For this review, take the finished solid that the model builds, in its own axes (mm). Face numbers are marked on the shaded views. A direction names the side the tool comes from. Coordinates: 2 decimals unless noted, no trailing zeros. Write each loop counter-clockwise with the first axis right and the second up, starting at its lowest first coordinate (ties: lowest second). Pieces come first, ordered by that corner, then holes. Notation, with made-up numbers: M 48,32.5 L 55,32.5 A25 cw 55,69.5 Z; hole C 41.5,-37.5 d7. An arc over 180 degrees is marked long. Return JSON: item names as keys, results as strings.
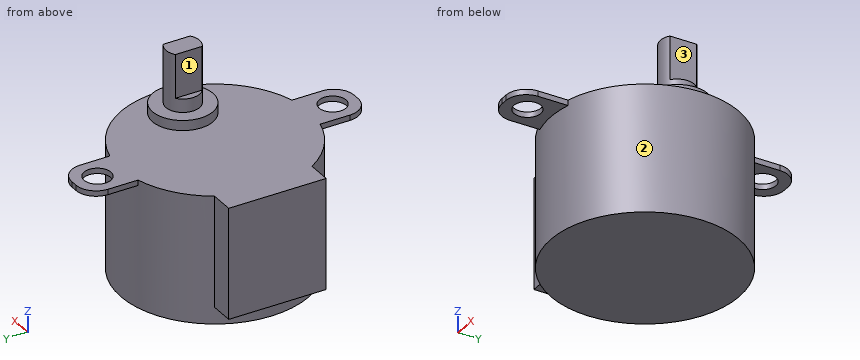
```python
from build123d import *

# Parameters (mm, degrees)
CYLINDER012_R             = 2
CYLINDER012_DEPTH         = 20
CYLINDER011_R             = 2
CYLINDER011_DEPTH         = 20
CYLINDER014_R             = 4.5
CYLINDER014_DEPTH         = 19.5
BOX009_W                  = 7
BOX009_H                  = 42
BOX009_DEPTH              = 0.8
FILLET008_R               = 3
FILLET009_R               = 3
FILLET010_R               = 3
FILLET011_R               = 3
BOX008_W                  = 10
BOX008_H                  = 14.5
BOX008_DEPTH              = 16.5
CYLINDER010_R             = 14
CYLINDER010_DEPTH         = 19
BOX010_W                  = 10
BOX010_H                  = 10
BOX010_DEPTH              = 10
BOX011_W                  = 10
BOX011_H                  = 10
BOX011_DEPTH              = 10
CYLINDER013_R             = 2.5
CYLINDER013_DEPTH         = 28
FUSION011_PLACEMENT_ANGLE = 180


with BuildPart() as cylinder012:
    # Cylinder012 → Cylinder012 (new body)
    with BuildSketch(Plane(origin=(0, -17.5, 14), x_dir=(1, 0, 0), z_dir=(0, 0, 1))):
        Circle(CYLINDER012_R)
    extrude(amount=CYLINDER012_DEPTH)


with BuildPart() as cylinder011:
    # Cylinder011 → Cylinder011 (new body)
    with BuildSketch(Plane(origin=(0, 17.5, 14), x_dir=(1, 0, 0), z_dir=(0, 0, 1))):
        Circle(CYLINDER011_R)
    extrude(amount=CYLINDER011_DEPTH)


with BuildPart() as shaft_boss002:
    # Cylinder014 → Cylinder014 (new body)
    with BuildSketch(Plane(origin=(-8, 0, 1), x_dir=(1, 0, 0), z_dir=(0, 0, 1))):
        Circle(CYLINDER014_R)
    extrude(amount=CYLINDER014_DEPTH)


with BuildPart() as fillet011:
    # Box009 → Box009 (new body)
    with BuildSketch(Plane(origin=(-3.5, -21, 18.2), x_dir=(1, 0, 0), z_dir=(0, 0, 1))):
        with Locations((3.5, 21)):
            Rectangle(BOX009_W, BOX009_H)
    extrude(amount=BOX009_DEPTH)

    # Fillet008
    fillet008_edges = [fillet011.edges().sort_by_distance(p)[0] for p in [
        (3.5, -21, 18.6),
    ]]
    fillet(fillet008_edges, radius=FILLET008_R)

    # Fillet009
    fillet009_edges = [fillet011.edges().sort_by_distance(p)[0] for p in [
        (-3.5, -21, 18.6),
    ]]
    fillet(fillet009_edges, radius=FILLET009_R)

    # Fillet010
    fillet010_edges = [fillet011.edges().sort_by_distance(p)[0] for p in [
        (-3.5, 21, 18.6),
    ]]
    fillet(fillet010_edges, radius=FILLET010_R)

    # Fillet011
    fillet011_edges = [fillet011.edges().sort_by_distance(p)[0] for p in [
        (3.5, 21, 18.6),
    ]]
    fillet(fillet011_edges, radius=FILLET011_R)


with BuildPart() as cube008:
    # Box008 → Box008 (new body)
    with BuildSketch(Plane(origin=(5.5, -7.25, 2.5), x_dir=(1, 0, 0), z_dir=(0, 0, 1))):
        with Locations((5, 7.25)):
            Rectangle(BOX008_W, BOX008_H)
    extrude(amount=BOX008_DEPTH)


with BuildPart() as motor_body002:
    # Cylinder010 → Cylinder010 (new body)
    with BuildSketch(Plane.XY):
        Circle(CYLINDER010_R)
    extrude(amount=CYLINDER010_DEPTH)

    # Fusion008: union Cube008
    add(cube008.part)

    # Fusion009: union Fillet011
    add(fillet011.part)

    # Fusion010: union shaft-boss002
    add(shaft_boss002.part)

    # Cut010: cut Cylinder011
    add(cylinder011.part, mode=Mode.SUBTRACT)

    # Cut011: cut Cylinder012
    add(cylinder012.part, mode=Mode.SUBTRACT)


with BuildPart() as cube010:
    # Box010 → Box010 (new body)
    with BuildSketch(Plane(origin=(-6.5, -5, 22.5), x_dir=(1, 0, 0), z_dir=(0, 0, 1))):
        with Locations((5, 5)):
            Rectangle(BOX010_W, BOX010_H)
    extrude(amount=BOX010_DEPTH)


with BuildPart() as cube011:
    # Box011 → Box011 (new body)
    with BuildSketch(Plane(origin=(-19.5, -5, 22.5), x_dir=(1, 0, 0), z_dir=(0, 0, 1))):
        with Locations((5, 5)):
            Rectangle(BOX011_W, BOX011_H)
    extrude(amount=BOX011_DEPTH)


with BuildPart() as obj1:
    # Cylinder013 → Cylinder013 (new body)
    with BuildSketch(Plane(origin=(-8, 0, 1), x_dir=(1, 0, 0), z_dir=(0, 0, 1))):
        Circle(CYLINDER013_R)
    extrude(amount=CYLINDER013_DEPTH)

    # Cut008: cut Cube011
    add(cube011.part, mode=Mode.SUBTRACT)

    # Cut009: cut Cube010
    add(cube010.part, mode=Mode.SUBTRACT)

    # Fusion011: union motor-body002
    add(motor_body002.part)


with BuildPart() as obj1_1:
    # Fusion011 placement: moved
    add(obj1.part.moved(Location((-8.1, 7, 7))).rotate(Axis((-8.1, 7, 7), (0, 0, 1)), FUSION011_PLACEMENT_ANGLE))


solid = obj1_1.part
```
1. We need section A-A (y = 24.5). State the section outline as (x, z) points.
Checks:
{"outline": "M -11.6,25.2 L -10.1,25.2 L -10.1,26 L -11.6,26 Z; M -6.1,25.2 L -4.6,25.2 L -4.6,26 L -6.1,26 Z"}
2. Clearance check with flat-ended pins moving along their axes: pin 1 Ø3 at (x, z) = (-22, 20.5) entering from -Y; pin 2 Ø8 at (y, z) = (-4.5, 32) entering from -X; pin 3 Ø0.5 at (x, y) = (-2, 7) entering from +Z; pin 4 Ø5 at (x, z) = (-14.5, 13) entering from +Y. State where each tip first meets the part, or that it passes through.
Checks:
{"pin 1": "y = -0.25", "pin 2": "through", "pin 3": "z = 29.5", "pin 4": "y = 20.45"}
3. We need section C-C (y = 7). State the section outline as (x, z) points, plus the area to 3 significant figures.
Checks:
{"outline": "M -23.6,9.5 L -22.1,9.5 L -22.1,7 L 5.9,7 L 5.9,26 L 4.4,26 L 4.4,27.5 L 2.4,27.5 L 2.4,29.5 L 1.4,29.5 L 1.4,36 L -1.6,36 L -1.6,29.5 L -2.6,29.5 L -2.6,27.5 L -4.6,27.5 L -4.6,26 L -23.6,26 Z", "area": "600 mm2"}
4. We need section D-D (z = 20.25). State the section outline as (x, y) points.
Checks:
{"outline": "M -23.6,-0.25 L -20.08,-0.25 A14 ccw long -20.08,14.25 L -23.6,14.25 Z"}
5. For the marked faces 1, 2 and 3, list the 3-axis set-ups (+Z, -Z, +X, -X, +Y, -Y) from which the entire face can be reached by the end or side of a thin tool; tool diameter is ignored.
Checks:
{"face 1": "+Z, -X, +Y, -Y", "face 2": "-Z", "face 3": "+Z, +X, +Y, -Y"}
6. We need section B-B (x = -8.1). State the section outline as (y, z) points.
Checks:
{"outline": "M -14,25.2 L -12.5,25.2 L -12.5,26 L -14,26 Z; M -8.5,25.2 L -7,25.2 L -7,7 L 21,7 L 21,25.2 L 22.5,25.2 L 22.5,26 L -8.5,26 Z; M 26.5,25.2 L 28,25.2 L 28,26 L 26.5,26 Z"}
7. Wall thickness on L1, parallel to Y at x = -8.1, z = 25.55; L2, parallel to Z at x = -6, y = 15.5; L3, parallel to Z at x = -22, y = 10.5: over which ranges is each line inside the solid? List them lowest first. Write a range as from..to.
Checks:
{"L1": "-14..-12.5, -8.5..22.5, 26.5..28", "L2": "7..26", "L3": "9.5..26"}
